```python
from build123d import *

# Parameters (mm, degrees)
F0_W     = 12.1363507145
F0_H     = 8.9991581862
F1_DEPTH = 10
F2_R     = 3.0408929123


with BuildPart() as f1:
    # F0 (on Right) → F1 (new body)
    with BuildSketch(Plane.YZ):
        Polygon((-14.7514826591, 1.1445179262), (-26.8878333736, 1.1445179262), (-26.8878333736, 1.1436761124), (3.1121666264, 1.1436761124), (3.1121666264, 10.1436761124), (-14.7514826591, 10.1436761124), align=None)
        with Locations((-20.8196580164, 5.6440970193)):
            Rectangle(F0_W, F0_H)
        Polygon((-44.7503355374, 1.1483416653), (-44.7514826591, 1.1445179262), (-26.8878333736, 1.1445179262), (-26.8878333736, 10.1436761124), (-14.7514826591, 10.1436761124), (-14.7514826591, 101.1445179262), (-42.5003355374, 8.6483416653), (-40.2435733936, 8.6483416653), (-40.2435733936, 1.1483416653), (-44.7435733936, 1.1483416653), align=None)
        Polygon((-48.7435733936, 1.1483416653), (-44.7503355374, 1.1483416653), (-44.7435733936, 1.1708821449), (-44.7435733936, 8.6483416653), (-44.7435733936, 16.1483416653), (-48.7435733936, 16.1483416653), align=None)
        Polygon((-44.7435733936, 8.6483416653), (-44.7435733936, 1.1708821449), (-42.5003355374, 8.6483416653), align=None)
        Polygon((-42.5003355374, 8.6483416653), (-44.7435733936, 1.1708821449), (-44.7435733936, 1.1483416653), (-40.2435733936, 1.1483416653), (-40.2435733936, 8.6483416653), align=None)
        Polygon((-44.7435733936, 1.1708821449), (-44.7503355374, 1.1483416653), (-44.7435733936, 1.1483416653), align=None)
    extrude(amount=F1_DEPTH)

    # F2
    f2_edges = [f1.edges().sort_by_distance(p)[0] for p in [
        (5, -14.751483, 101.144518),
    ]]
    fillet(f2_edges, radius=F2_R)


solid = f1.part
```
Geometry check sheet. Reference: the model listing, model coordinates, mm. A direction names the side the tool comes from. Give positions to 0.01 mm unless a question says otherwise; leave off trailing zeros. Write each loop counter-clockwise with the first axis right and the second up, starting at its lowest first coordinate (ties: lowest second). Pieces come first, ordered by that corner, then holes. Notation, with made-up numbers: (30, -35) - (46, -35) arc R3 ccw to (46, -30) - close; hole circle Ø6 at (-9.75, -30). An arc over 180 degrees is marked (long way). Use a Markdown table: item, result.
Q1. Section check B-B, the plane y = -10. Enter the section's corners in (x, z).
Computed:
| item | result |
|---|---|
| outline | (0, 1.14) - (10, 1.14) - (10, 10.14) - (0, 10.14) - close |
Q2. Draft check along Y on faces 1 (the face through (5, -44.744, 12)), 2 (the face through (5, -48.744, 9)), 3 (the face through (5, -12, 1.144)). Enter one of: pulls with the +Y half, pulls with the -Y half, needs draft (parallel to the pull), parting line crosses it, or undercut.
Computed:
| item | result |
|---|---|
| face 1 | undercut |
| face 2 | pulls with the -Y half |
| face 3 | needs draft |
Q3. Section check C-C, the plane z = 54.5. Enter the section's corners in (x, y).
Computed:
| item | result |
|---|---|
| outline | (0, -28.74) - (10, -28.74) - (10, -14.75) - (0, -14.75) - close |
Q4. Thickness scan on L1, parallel to Z at x = 3, y = -11; L2, parallel to Z at x = 8.5, y = -43; L3, parallel to Y at x = 9.5, z = 68. Record the ranges inside material, lowest first. Write a range as [from, to].
Computed:
| item | result |
|---|---|
| L1 | z = [1.14, 10.14] |
| L2 | z = [1.14, 8.65] |
| L3 | y = [-24.69, -14.75] |
Q5. Go/stop test with flat-tipped pins: P1, Ø1.2, axis at x = 7, y = -47, coming from the -Z side; P2, Ø1.2, axis at x = 2.5, y = -46, coming from the +Z side; P3, Ø6, axis at x = 4.5, z = 64, coming from the -Y side. Record where each tip stops, or that it passes through.
Computed:
| item | result |
|---|---|
| P1 | stops at z = 1.15 |
| P2 | stops at z = 16.15 |
| P3 | stops at y = -26.79 |
Q6. Set-up check for faces 4 (the face through (5, -44, 8.648)), 5 (the face through (5, -14.751, 45)), 6 (the face through (5, -47, 1.148)), 7 (the face through (5, 3.112, 6)), 8 (the face through (5, -47, 16.148)): record each of +Z, -Z, +X, -X, +Y, -Y from which the full face is reachable in a straight line by a thin tool's end or side.
Computed:
| item | result |
|---|---|
| face 4 | +Z, +X, -X |
| face 5 | +Z, +X, -X, +Y |
| face 6 | -Z, +X, -X, +Y, -Y |
| face 7 | +Z, -Z, +X, -X, +Y |
| face 8 | +Z, +X, -X, -Y |
